from build123d import *

# Parameters (mm, degrees)
SKETCH1_W                = 13
SKETCH1_H                = 67
BOSS_EXTRUDE1_DEPTH      = 30
SKETCH2_W                = 67.456445976
SKETCH2_H                = 61
CUT_EXTRUDE1_DEPTH       = 10
M4_CLEARANCE_HOLE3_D     = 4.5
M4_CLEARANCE_HOLE3_DEPTH = 6
M4_CLEARANCE_HOLE3_TIP   = 1.351936393
M4_CLEARANCE_HOLE1_D     = 4.5
M4_CLEARANCE_HOLE1_DEPTH = 6
M4_CLEARANCE_HOLE1_TIP   = 1.351936393
M4_CLEARANCE_HOLE2_D     = 4.5
M4_CLEARANCE_HOLE2_DEPTH = 6
M4_CLEARANCE_HOLE2_TIP   = 1.351936393


with BuildPart() as part:
    # Sketch1 → Boss-Extrude1 (new body)
    with BuildSketch(Plane.XY):
        Rectangle(SKETCH1_W, SKETCH1_H)
    extrude(amount=BOSS_EXTRUDE1_DEPTH)

    # Sketch2 → Cut-Extrude1 (cut)
    with BuildSketch(Plane(origin=(6.5, 0, 0), x_dir=(0, 0, -1), z_dir=(1, 0, 0))):
        with Locations((-11.6230653, 0)):
            Rectangle(SKETCH2_W, SKETCH2_H)
    extrude(amount=-CUT_EXTRUDE1_DEPTH, mode=Mode.SUBTRACT)

    # M4 Clearance Hole3
    with Locations(Plane(origin=(0, 33.5, 0), x_dir=(1, 0, 0), z_dir=(0, 1, 0))):
        with Locations((0.724225785, -12.024273001)):
            Hole(M4_CLEARANCE_HOLE3_D / 2, depth=M4_CLEARANCE_HOLE3_DEPTH)
            with Locations((0, 0, -(M4_CLEARANCE_HOLE3_DEPTH + M4_CLEARANCE_HOLE3_TIP / 2))):  # 118° drill point
                Cone(0, M4_CLEARANCE_HOLE3_D / 2, M4_CLEARANCE_HOLE3_TIP, mode=Mode.SUBTRACT)

    # M4 Clearance Hole1
    with Locations(Plane(origin=(0, -30.5, 0), x_dir=(1, 0, 0), z_dir=(0, 1, 0))):
        with Locations((1.5, -5.008015198), (1.5, -24.910664678)):
            Hole(M4_CLEARANCE_HOLE1_D / 2, depth=M4_CLEARANCE_HOLE1_DEPTH)
            with Locations((0, 0, -(M4_CLEARANCE_HOLE1_DEPTH + M4_CLEARANCE_HOLE1_TIP / 2))):  # 118° drill point
                Cone(0, M4_CLEARANCE_HOLE1_D / 2, M4_CLEARANCE_HOLE1_TIP, mode=Mode.SUBTRACT)

    # M4 Clearance Hole2
    with Locations(Plane(origin=(0, 33.5, 0), x_dir=(1, 0, 0), z_dir=(0, 1, 0))):
        with Locations((0.958202429, -17.944695077)):
            Hole(M4_CLEARANCE_HOLE2_D / 2, depth=M4_CLEARANCE_HOLE2_DEPTH)
            with Locations((0, 0, -(M4_CLEARANCE_HOLE2_DEPTH + M4_CLEARANCE_HOLE2_TIP / 2))):  # 118° drill point
                Cone(0, M4_CLEARANCE_HOLE2_D / 2, M4_CLEARANCE_HOLE2_TIP, mode=Mode.SUBTRACT)


solid = part.part
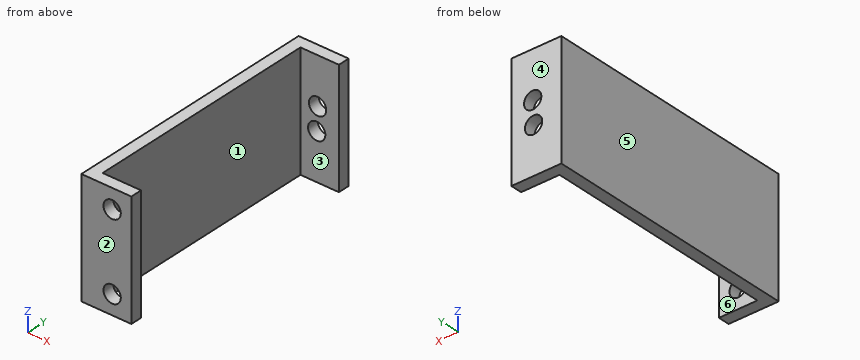
Geometry: final body of the model. Coordinates: model frame, mm. Face numbers are marked on the shaded views. A direction names the side the tool comes from. Give positions to 0.01 mm unless a question says otherwise; leave off trailing zeros. Loops run counter-clockwise (first coordinate to the right, second up) from the corner with the lowest first, then second, coordinate; pieces in that order, holes last. Notation, with made-up numbers: (60.5, 37) - (89.5, 37) arc R18 ccw to (89.5, 51) - close; hole circle Ø2 at (40.5, 41.25). An arc over 180 degrees is marked (long way). Answer as CSV lines item,"result". Start each with the question number.
1. Reachability of the marked faces 1 and 2 from +Z, -Z, +X, -X, +Y, -Y: full face, straight path, thin tool, end or side. Return the list, or none.
2. Pin query (flat end, axial travel): P1, Ø3.5, axis at x = 1.5, z = 5.01, coming from the -Y side; P2, Ø15, axis at y = 13.5, z = 21, coming from the +X side. Return the tip coordinate at first contact, or that it passes through.
3. Draft query along Y for the marked faces 3, 4, 5 and 6. Return one class per face: released by +Y, released by -Y, zero draft, split by the parting line, or undercut.
4. Section A-A, the plane x = 1.5. Return loops of the section in (y, z).
5. Ray query, L1, parallel to Z at x = 1.5, y = -31.2; L2, parallel to Y at x = 2, z = 22.5; L3, parallel to X at y = 16, z = 20. Return the intervals inside material, ascending.
6. Section B-B, the plane z = 5.75. Return loops of the section in (x, y).
7. Section C-C, the plane y = 17. Return loops of the section in (x, z).
Answers:
1,face 1,"+Z, -Z, +X"
1,face 2,"+Z, -Z, +X, -X, -Y"
2,P1,"stops at y = 30.5"
2,P2,"stops at x = -3.5"
3,face 3,"undercut"
3,face 4,"released by +Y"
3,face 5,"zero draft"
3,face 6,"undercut"
4,outline,"(-33.5, 0) - (-30.5, 0) - (-30.5, 2.76) - (-33.5, 2.76) - close; (-33.5, 7.26) - (-30.5, 7.26) - (-30.5, 22.66) - (-33.5, 22.66) - close; (-33.5, 27.16) - (-30.5, 27.16) - (-30.5, 30) - (-33.5, 30) - close; (30.5, 0) - (33.5, 0) - (33.5, 9.91) - (30.5, 9.91) - close; (30.5, 14.14) - (33.5, 14.14) - (33.5, 15.76) - (30.5, 15.76) - close; (30.5, 20.13) - (33.5, 20.13) - (33.5, 30) - (30.5, 30) - close"
5,L1,"z = 0 to 2.76, 7.26 to 22.66, 27.16 to 30"
5,L2,"y = -33.5 to -30.5, 30.5 to 33.5"
5,L3,"x = -6.5 to -3.5"
6,outline,"(-6.5, -33.5) - (-0.62, -33.5) - (-0.62, -30.5) - (-3.5, -30.5) - (-3.5, 30.5) - (6.5, 30.5) - (6.5, 33.5) - (-6.5, 33.5) - close; (3.62, -33.5) - (6.5, -33.5) - (6.5, -30.5) - (3.62, -30.5) - close"
7,outline,"(-6.5, 0) - (-3.5, 0) - (-3.5, 30) - (-6.5, 30) - close"
